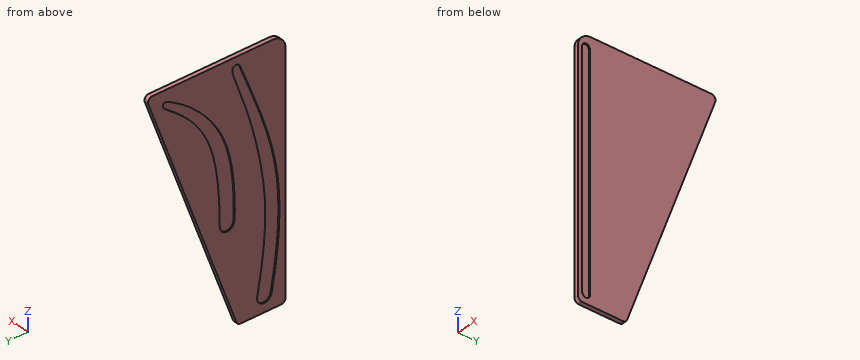
from build123d import *

# Parameters (mm, degrees)
BOSS_EXTRUDE1_DEPTH = 10
CUT_EXTRUDE4_DEPTH  = 3
CUT_EXTRUDE5_DEPTH  = 3


with BuildPart() as part:
    # Sketch1 → Boss-Extrude1 (new body)
    with BuildSketch(Plane(origin=(0, 0, 0), x_dir=(0, 0, -1), z_dir=(1, 0, 0))):
        with BuildLine():
            Line((0, -14.281480067), (0, -294.281480067))
            ThreePointArc((0, -294.281480067), (8.786796564, -315.494683503), (30, -324.281480067))
            Line((30, -324.281480067), (573.815572472, -324.281480067))
            ThreePointArc((573.815572472, -324.281480067), (580.886640283, -321.352547879), (583.815572472, -314.281480067))
            Line((583.815572472, -314.281480067), (583.815572472, -219.493566063))
            ThreePointArc((583.815572472, -219.493566063), (582.007092914, -213.757801699), (577.235773905, -210.096639855))
            Line((577.235773905, -210.096639855), (13.420201433, -4.88455386))
            ThreePointArc((13.420201433, -4.88455386), (4.264235636, -6.089959625), (0, -14.281480067))
        make_face()
    extrude(amount=BOSS_EXTRUDE1_DEPTH)

    # Sketch3 → Cut-Extrude4 (cut)
    with BuildSketch(Plane.ZY):
        with BuildLine():
            ThreePointArc((-23.162175785, -218.017297737), (-17.576945532, -207.678107035), (-26.738120061, -200.318314743))
            add(Edge.make_bspline(
                [(-26.738120061, -200.318314743), (-45.914354434, -200.660753587), (-151.32107334, -255.510398156), (-414.880335601, -286.385074175), (-542.431128002, -257.731725159), (-546.154906269, -257.731029979)],
                knots=[0, 0, 0, 0, 0.560935224, 0.660935224, 1, 1, 1, 1], degree=3))
            ThreePointArc((-546.154906269, -257.731029979), (-563.288388976, -273.27487263), (-549.474047026, -291.831036849))
            add(Edge.make_bspline(
                [(-549.474047026, -291.831036849), (-474.750080899, -306.502271197), (-284.669923623, -324.572171749), (-143.080818041, -266.034178467), (-23.162175785, -218.017297737)],
                knots=[0, 0, 0, 0, 0.423888314, 1, 1, 1, 1], degree=3))
        make_face()
        with BuildLine():
            ThreePointArc((-26.950185671, -47.737214996), (-28.17113687, -40.715672082), (-35.124917897, -39.154353359))
            add(Edge.make_bspline(
                [(-35.124917897, -39.154353359), (-50.602952828, -45.122445935), (-99.042539, -170.661871263), (-331.224003862, -171.181746235), (-353.169530365, -171.181734297)],
                knots=[0, 0, 0, 0, 0.639195597, 1, 1, 1, 1], degree=3))
            ThreePointArc((-353.169530365, -171.181734297), (-370.309371751, -186.812434708), (-356.32010769, -205.316311305))
            add(Edge.make_bspline(
                [(-356.32010769, -205.316311305), (-352.838937223, -205.964445921), (-121.396454164, -217.989087479), (-35.312726243, -66.629555086), (-26.950185671, -47.737214996)],
                knots=[0, 0, 0, 0, 0.40968467, 1, 1, 1, 1], degree=3))
        make_face()
    extrude(amount=-CUT_EXTRUDE4_DEPTH, mode=Mode.SUBTRACT)

    # Sketch5 → Cut-Extrude5 (cut)
    with BuildSketch(Plane(origin=(10, 0, 0), x_dir=(0, 0, -1), z_dir=(1, 0, 0))):
        with BuildLine():
            Line((561.587294138, -296.630106089), (27.291979273, -296.630106089))
            ThreePointArc((27.291979273, -296.630106089), (18.291979273, -305.630106089), (27.291979273, -314.630106089))
            Line((27.291979273, -314.630106089), (561.587294138, -314.630106089))
            ThreePointArc((561.587294138, -314.630106089), (570.587294138, -305.630106089), (561.587294138, -296.630106089))
        make_face()
    extrude(amount=-CUT_EXTRUDE5_DEPTH, mode=Mode.SUBTRACT)


solid = part.part
Geometry check sheet. Reference: the model listing, model coordinates, mm. Give positions to 0.01 mm unless a question says otherwise; leave off trailing zeros. Order: outer loops, then holes, each group sorted by start corner. A loop starts at its lowest first (then second) coordinate and runs counter-clockwise, first axis right, second up.
1. Scan lines: line 1 (Y direction, x = 0.5, z = -181.5); line 2 (X direction, y = -297, z = -244); line 3 (Y direction, x = 8.5, z = -75). Record each from-to range of solid material in increasing order.
Completed:
line 1: y = -324.28 to -278.07, -249.57 to -186.36, -152.77 to -66.06
line 2: x = 0 to 7
line 3: y = -324.28 to -314.63, -296.63 to -27.3
2. Sectioned sample at B-B (y = -26). Record the boundary of the cut face in (x, z), then the cut area to 3 significant figures.
Completed:
outline: (0, -71.43) - (10, -71.43) - (10, 0) - (0, 0) - close
area: 714 mm2
3. Sectioned sample at A-A (x = 5). Record the boundary of the cut face in (y, z).
Completed:
outline: (-324.28, -573.82) arc R10 ccw to (-314.28, -583.82) - (-219.49, -583.82) arc R10 ccw to (-210.1, -577.24) - (-4.88, -13.42) arc R10 ccw to (-14.28, 0) - (-294.28, 0) arc R30 ccw to (-324.28, -30) - close
4. Depth check by flat-ended pin: pin 1 (9 mm diameter, centred on y = -301.5, z = -278.5, fed in from +X); pin 2 (0.9 mm diameter, centred on x = 9, z = -217.5, fed in from +Y); pin 3 (1.5 mm diameter, centred on x = 5, z = -141.5, fed in from +Y). Enter the tip coordinate at first touch or a pass-through.
Completed:
pin 1: stops at x = 7
pin 2: stops at y = -79
pin 3: stops at y = -51.23
